```python
from build123d import *

# Parameters (mm, degrees)
SKETCH1_R               = 8
BOSS_EXTRUDE1_DEPTH     = 20
SKETCH2_R               = 20
BOSS_EXTRUDE2_DEPTH     = 139
SKETCH3_R               = 15
CUT_EXTRUDE1_DEPTH      = 42
CUT_EXTRUDE1_DEPTH_BACK = 57
SKETCH4_W               = 4
SKETCH4_H               = 2.5
SKETCH5_R               = 16
CUT_EXTRUDE2_DEPTH      = 45.4
SKETCH6_R               = 9.5
CUT_EXTRUDE3_DEPTH      = 12
CHAMFER1_SIZE           = 2
FILLET1_R               = 3


with BuildPart() as part:
    # Sketch1 → Boss-Extrude1 (new body)
    with BuildSketch(Plane.XY):
        with BuildLine():
            Line((-56, 30), (41, 30))
            Line((41, 30), (41, 8))
            ThreePointArc((41, 8), (33, 0), (41, -8))
            Line((41, -8), (41, -40))
            Line((41, -40), (-56, -40))
            Line((-56, -40), (-56, 30))
        make_face()
        with Locations((-41, 0)):
            Circle(SKETCH1_R, mode=Mode.SUBTRACT)
    extrude(amount=BOSS_EXTRUDE1_DEPTH)

    # Sketch2 → Boss-Extrude2 (add)
    with BuildSketch(Plane.XY.offset(20)):
        Circle(SKETCH2_R)
    extrude(amount=BOSS_EXTRUDE2_DEPTH)

    # Sketch3 → Cut-Extrude1 (cut, two sides)
    with BuildSketch(Plane(origin=(0, 0, 0), x_dir=(0, 0, -1), z_dir=(1, 0, 0))) as cut_extrude1_sk:
        with Locations((-90, 0)):
            Circle(SKETCH3_R)
    extrude(amount=CUT_EXTRUDE1_DEPTH, mode=Mode.SUBTRACT)
    extrude(cut_extrude1_sk.sketch, amount=-CUT_EXTRUDE1_DEPTH_BACK, mode=Mode.SUBTRACT)

    # Sketch4 → Cut-Revolve1 (revolve, cut)
    with BuildSketch(Plane(origin=(0, 0, 0), x_dir=(0, 0, -1), z_dir=(1, 0, 0))):
        with Locations((-64, 18.75)):
            Rectangle(SKETCH4_W, SKETCH4_H)
        with Locations((-72, 18.75)):
            Rectangle(SKETCH4_W, SKETCH4_H)
        with Locations((-118.6, 18.75)):
            Rectangle(SKETCH4_W, SKETCH4_H)
    revolve(axis=Axis((0, 0, 0), (0, 0, 1)), mode=Mode.SUBTRACT)

    # Sketch5 → Cut-Extrude2 (cut)
    with BuildSketch(Plane.XY.offset(159)):
        Circle(SKETCH5_R)
    extrude(amount=-CUT_EXTRUDE2_DEPTH, mode=Mode.SUBTRACT)

    # Sketch6 → Cut-Extrude3 (cut)
    with BuildSketch(Plane.XY.offset(113.6)):
        Circle(SKETCH6_R)
    extrude(amount=-CUT_EXTRUDE3_DEPTH, mode=Mode.SUBTRACT)

    # Chamfer1
    chamfer1_edges = [part.edges().sort_by_distance(p)[0] for p in [
        (-20, 0, 159),
    ]]
    chamfer(chamfer1_edges, length=CHAMFER1_SIZE)

    # Fillet1
    fillet1_edges = [part.edges().sort_by_distance(p)[0] for p in [
        (-56, 30, 10),
        (-56, -40, 10),
        (-7.5, 30, 0),
        (-7.5, -40, 0),
    ]]
    fillet(fillet1_edges, radius=FILLET1_R)


solid = part.part
```
Build history of the part. All positions in model axes, mm. A direction names the side the tool comes from. Give positions to 0.01 mm unless a question says otherwise; leave off trailing zeros. Order: outer loops, then holes, each group sorted by start corner. A loop starts at its lowest first (then second) coordinate and runs counter-clockwise, first axis right, second up. Notation, with made-up numbers: M 13,-40 L 62,-40 A15 ccw 62,-14 Z; hole C 7,81 d1. An arc over 180 degrees is marked long. Return JSON: item names as keys, results as strings.
Q1. Wall check: probe 1 along Z at (x, y) = (33, 26); probe 2 along Z at (x, y) = (15.75, 0); probe 3 along Y at (x, z) = (-46.5, 16). Give the ranges that are in metal, low to high. Write a range as from..to.
Answer list:
{"probe 1": "z = 0..20", "probe 2": "z = 0..75, 105..113.6", "probe 3": "y = -40..-5.81, 5.81..30"}
Q2. Band-saw the part on C-C (y = 0). Count the separate pieces of the cut face and the enclosed holes in it, then the cut area to 3 significant figures.
Answer list:
{"separate pieces": "4", "enclosed holes": "0", "area": "4,140 mm^2"}
Q3. Flat gauge pins, fed straight in: pin 1 (4 mm diameter, centred on x = -8.5, z = 33, fed in from +Y); pin 2 (6 mm diameter, centred on x = -4, y = 2, fed in from +Z); pin 3 (6 mm diameter, centred on x = 21, z = 73.5, fed in from -Y). Where does each tip first touch, or does it go through?
Answer list:
{"pin 1": "stops at y = 18.91", "pin 2": "stops at z = 75.86", "pin 3": "stops at y = -8.63"}
Q4. Band-saw the part on A-A (x = -41). Give the cut face in (y, z).
Answer list:
{"outline": "M -40,3 A3 ccw -37,0 L -8,0 L -8,20 L -40,20 Z; M 8,0 L 27,0 A3 ccw 30,3 L 30,20 L 8,20 Z"}
Q5. Two-plate mould, pull along Y, no slides. Class faces 4 (the face through (18, 0, 62)), 5 (the face through (-55.1, 29.14, 10.14)), 6 (the face through (33, 0, 10)): pulls with the +Y half, pulls with the -Y half, needs draft (parallel to the pull), parting line crosses it, or undercut.
Answer list:
{"face 4": "needs draft", "face 5": "pulls with the +Y half", "face 6": "undercut"}
Q6. 3-axis set-ups, long thin cutter, end or side, ignore diameter. For faces 1 (the face through (10.648, -13.887, 118.572)), 2 (the face through (18.475, -7.66, 40.706)), 3 (the face through (41, -24, 10)): which of +Z, -Z, +X, -X, +Y, -Y reach the whole face in a straight line?
Answer list:
{"face 1": "none", "face 2": "+Z", "face 3": "+Z, -Z, +X, +Y, -Y"}
Q7. Band-saw the part on B-B (z = 16.5). Give the cut face in (x, y), then the cut area to 3 significant figures.
Answer list:
{"outline": "M -56,-37 A3 ccw -53,-40 L 41,-40 L 41,-8 A8 cw 41,8 L 41,30 L -53,30 A3 ccw -56,27 Z; hole C -41,0 d16", "area": "6,480 mm^2"}
Q8. Band-saw the part on D-D (z = 90). Give the cut face in (x, y), then the cut area to 3 significant figures.
Answer list:
{"outline": "M -13.23,-15 A20 ccw 13.23,-15 Z; M -13.23,15 L 13.23,15 A20 ccw Z", "area": "181 mm^2"}
